The drawing under review shows one solid part. Ordinate dimensions are in mm from its lowest x, y, z. A direction names the side the tool comes from. Give positions to 0.01 mm unless a question says otherwise; leave off trailing zeros. Order: outer loops, then holes, each group sorted by start corner. A loop starts at its lowest first (then second) coordinate and runs counter-clockwise, first axis right, second up. Notation, with made-up numbers: (14.5, 70.25) -> (59.5, 70.25) arc R14 ccw to (59.5, 95.25) -> close; hole circle Ø3 at (-31.75, 39.25). An arc over 180 degrees is marked (long way). Return JSON: item names as keys, results as strings. Group by question number.
1) For the marked faces 1 and 2, list the 3-axis set-ups (+Z, -Z, +X, -X, +Y, -Y) from which the entire face can be reached by the end or side of a thin tool; tool diameter is ignored.
2) To check wall thickness, follow line 1 along Z through (x, y) = (10, 9.5); line 2 along X through (y, z) = (1.3, 18.5). State the ranges of each line that lie inside material, in increasing order.
3) Add section C-C (y = 7.75). Give the boundary of the cut face in (x, z).
4) The part is to be moulded in two halves that separate along X. For the marked faces 3, 4 and 5, say which applies: released by +X, released by -X, zero draft, split by the parting line, or undercut.
5) Add section D-D (z = 18.5). Give the boundary of the cut face in (x, y), then the cut area to 3 significant figures.
6) Add section A-A (z = 10). Give the boundary of the cut face in (x, y), then the cut area to 3 significant figures.
7) Insertion check: P1, Ø1.6, axis at x = 18.5, z = 18.5, coming from the -Y side; P2, Ø6, axis at x = 3, z = 17.5, coming from the +Y side; P3, Ø5, axis at x = 3.5, y = 13, coming from the -Z side; P4, Ø3, axis at y = 13.5, z = 13, coming from the +X side. Each pin has a flat end and moves straight along its axis. Give the tip position at first contact, or say it passes through.
8) Add section B-B (x = 1.5). Give the boundary of the cut face in (y, z), then the cut area to 3 significant figures.
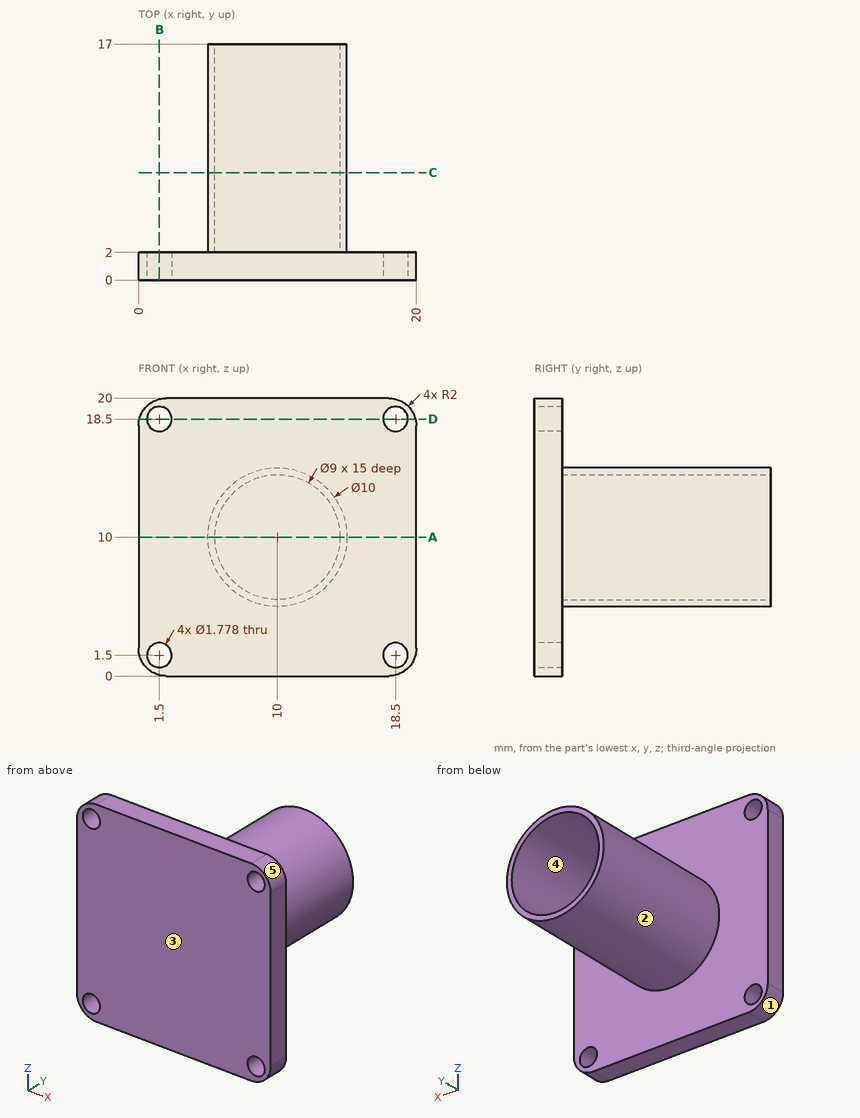
Evaluation:
{
 "1": {"face 1": "-Z, -X, +Y, -Y", "face 2": "+Y"},
 "2": {"line 1": "5 to 5.5, 14.5 to 15", "line 2": "0.06 to 0.61, 2.39 to 17.61, 19.39 to 19.94"},
 "3": {"outline": "circle Ø10 at (10, 10); hole circle Ø9 at (10, 10)"},
 "4": {"face 3": "zero draft", "face 4": "undercut", "face 5": "released by +X"},
 "5": {"outline": "(0.06, 0) -> (0.61, 0) -> (0.61, 2) -> (0.06, 2) -> close; (2.39, 0) -> (17.61, 0) -> (17.61, 2) -> (2.39, 2) -> close; (19.39, 0) -> (19.94, 0) -> (19.94, 2) -> (19.39, 2) -> close", "area": "32.6 mm^2"},
 "6": {"outline": "(0, 0) -> (20, 0) -> (20, 2) -> (15, 2) -> (15, 17) -> (14.5, 17) -> (14.5, 2) -> (5.5, 2) -> (5.5, 17) -> (5, 17) -> (5, 2) -> (0, 2) -> close", "area": "55.0 mm^2"},
 "7": {"P1": "through", "P2": "y = 2", "P3": "z = 7", "P4": "x = 14.77"},
 "8": {"outline": "(0, 0.06) -> (2, 0.06) -> (2, 0.61) -> (0, 0.61) -> close; (0, 2.39) -> (2, 2.39) -> (2, 17.61) -> (0, 17.61) -> close; (0, 19.39) -> (2, 19.39) -> (2, 19.94) -> (0, 19.94) -> close", "area": "32.6 mm^2"}
}
